Design review of the part shown in the three views and the two pictorial views. Dimensions are in mm from the part's minimum x, y and z. Coordinates: 2 decimals unless noted, no trailing zeros. Loops run counter-clockwise (first coordinate to the right, second up) from the corner with the lowest first, then second, coordinate; pieces in that order, holes last. Notation, with made-up numbers: (84, -24.75) -> (92, -24.75) arc R24 ccw to (92, -13.75) -> close; hole circle Ø10 at (-26.5, 12.25). An arc over 180 degrees is marked (long way). One line per item, written item: value.
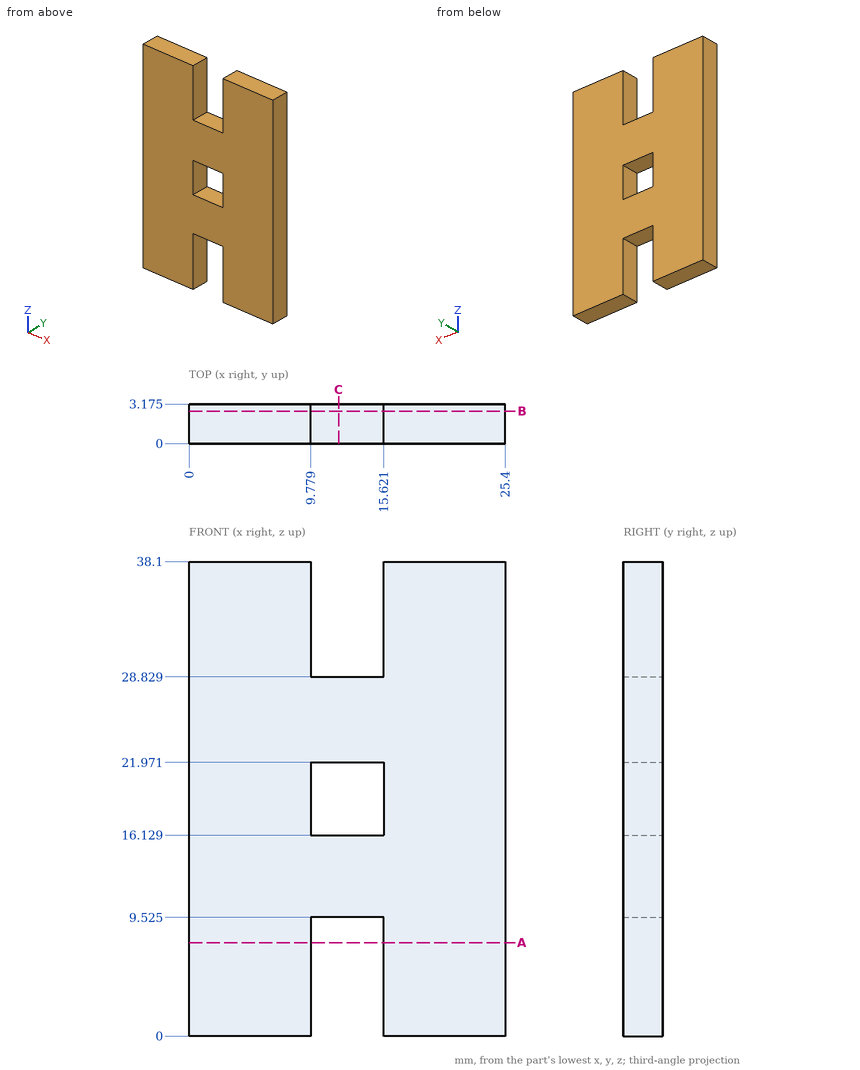
1. To check wall thickness, follow probe 1 along X at (y, z) = (2.6, 5); probe 2 along Z at (x, y) = (12.5, 0.75) (3 decimals). State the ranges of each line that lie inside material, in increasing order. Write a range as from..to.
Return value:
probe 1: x = 0..9.78, 15.62..25.4
probe 2: z = 9.525..16.129, 21.971..28.829
2. Take a section at A-A, the plane z = 7.5. Give the boundary of the cut face in (x, y) (3 decimals), and give its area (3 significant figures).
Return value:
outline: (0, 0) -> (9.779, 0) -> (9.779, 3.175) -> (0, 3.175) -> close; (15.621, 0) -> (25.4, 0) -> (25.4, 3.175) -> (15.621, 3.175) -> close
area: 62.1 mm2
3. Take a section at C-C, the plane x = 12. Give the boundary of the cut face in (y, z) (3 decimals).
Return value:
outline: (0, 9.525) -> (3.175, 9.525) -> (3.175, 16.129) -> (0, 16.129) -> close; (0, 21.971) -> (3.175, 21.971) -> (3.175, 28.829) -> (0, 28.829) -> close
4. Insertion check: pin 1 Ø1.6 at (x, y) = (11.5, 1) entering from +Z; pin 2 Ø1.6 at (x, y) = (13, 1.5) entering from -Z (3 decimals). Each pin has a flat end and moves straight along its axis. Give the tip position at first contact, or say it passes through.
Return value:
pin 1: stops at z = 28.83
pin 2: stops at z = 9.525
5. Take a section at B-B, the plane y = 2.6. Give the boundary of the cut face in (x, z) (3 decimals).
Return value:
outline: (0, 0) -> (9.779, 0) -> (9.779, 9.525) -> (15.621, 9.525) -> (15.621, 0) -> (25.4, 0) -> (25.4, 38.1) -> (15.621, 38.1) -> (15.621, 28.829) -> (9.779, 28.829) -> (9.779, 38.1) -> (0, 38.1) -> close; hole (9.779, 16.129) -> (15.621, 16.129) -> (15.621, 21.971) -> (9.779, 21.971) -> close
